```python
from build123d import *

# Parameters (mm, degrees)
F0_W         = 90
F0_H         = 11
F0_R         = 1.725
F0_R_2       = 1.7
F1_DEPTH     = 13
F2_R         = 5
F2_R_2       = 1.7
F3_DEPTH     = 24
F4_R         = 1.725
F5_DEPTH     = 24
F6_R         = 0.5
F7_DEPTH     = 12
F8_T1_DEPTH  = 28
F8_T6_DEPTH  = 105
F8_S7_R      = 5
F8_T8_DEPTH  = 54
F8_S9_R      = 5
F8_T10_DEPTH = 54
F8_T14_DEPTH = 105
F8_S15_R     = 5
F8_T16_DEPTH = 54
F8_S17_R     = 5
F8_T18_DEPTH = 54


# Not quite as in the source:
# - a fillet or chamfer that OpenCascade refuses, or shapes differently, is made with other operations: its cross-section is extruded or revolved along the edge and cut away or added
# - a feature names something its author has since deleted; it is built from what else it names


with BuildPart() as f1:
    # F0 (on Top) → F1 (new body)
    with BuildSketch(Plane.XY):
        Rectangle(F0_W, F0_H)
        with Locations((-40, 0)):
            Circle(F0_R, mode=Mode.SUBTRACT)
        with Locations((40, 0)):
            Circle(F0_R_2, mode=Mode.SUBTRACT)
    extrude(amount=F1_DEPTH)

    # F2 (on face) → F3 (join)
    with BuildSketch(Plane.XY.offset(13)):
        with Locations((40, 0)):
            Circle(F2_R)
        with Locations((40, 0)):
            Circle(F2_R_2, mode=Mode.SUBTRACT)
    extrude(amount=F3_DEPTH)

    # F4 (on face) → F5 (join)
    with BuildSketch(Plane.XY.offset(13)):
        with BuildLine():
            ThreePointArc((-45, 0), (-40, -5), (-35, 0))
            ThreePointArc((-35, 0), (-40, 5), (-45, 0))
        make_face()
        with Locations((-40, 0)):
            Circle(F4_R, mode=Mode.SUBTRACT)
    extrude(amount=F5_DEPTH)

    # F6 (on face) → F7 (cut)
    with BuildSketch(Plane.XY.offset(13)):
        with Locations((-20, 0)):
            Circle(F6_R)
        with Locations((20, 0)):
            Circle(F6_R)
    extrude(amount=-F7_DEPTH, mode=Mode.SUBTRACT)

    # F8: fillet of radius 3 on 6 edges, made by hand

    # F8_s2 → F8_t1 (cut)
    with BuildSketch(Plane.XY.offset(-7.5)):
        with BuildLine():
            ThreePointArc((-42, -5.5), (-44.1213203436, -4.6213203436), (-45, -2.5))
            Line((-45, -2.5), (-45, -5.5))
            Line((-45, -5.5), (-42, -5.5))
        make_face()
        with BuildLine():
            ThreePointArc((-45, 2.5), (-44.1213203436, 4.6213203436), (-42, 5.5))
            Line((-42, 5.5), (-45, 5.5))
            Line((-45, 5.5), (-45, 2.5))
        make_face()
        with BuildLine():
            ThreePointArc((42, -5.5), (44.1213203436, -4.6213203436), (45, -2.5))
            Line((45, -2.5), (45, -5.5))
            Line((45, -5.5), (42, -5.5))
        make_face()
        with BuildLine():
            ThreePointArc((45, 2.5), (44.1213203436, 4.6213203436), (42, 5.5))
            Line((42, 5.5), (45, 5.5))
            Line((45, 5.5), (45, 2.5))
        make_face()
    extrude(amount=F8_T1_DEPTH, mode=Mode.SUBTRACT)


with BuildPart() as f8_tool4:
    # F8_s5 → F8_t6 (new body)
    with BuildSketch(Plane.YZ.offset(-52.5)):
        with BuildLine():
            ThreePointArc((-5.5, 10), (-4.6213203436, 12.1213203436), (-2.5, 13))
            Line((-2.5, 13), (-5.5, 13))
            Line((-5.5, 13), (-5.5, 10))
        make_face()
    extrude(amount=F8_T6_DEPTH)

    # F8_s7 → F8_t8 (cut, symmetric)
    with BuildSketch(Plane.XY.offset(11.5)):
        with Locations((-40, 0)):
            Circle(F8_S7_R)
    extrude(amount=F8_T8_DEPTH, both=True, mode=Mode.SUBTRACT)

    # F8_s9 → F8_t10 (cut, symmetric)
    with BuildSketch(Plane.XY.offset(11.5)):
        with Locations((40, 0)):
            Circle(F8_S9_R)
    extrude(amount=F8_T10_DEPTH, both=True, mode=Mode.SUBTRACT)


with BuildPart() as f1_1:
    add(f1.part)

    # F8_t3: cut F8_tool4
    add(f8_tool4.part, mode=Mode.SUBTRACT)


with BuildPart() as f8_tool12:
    # F8_s13 → F8_t14 (new body)
    with BuildSketch(Plane.YZ.offset(52.5)):
        with BuildLine():
            ThreePointArc((2.5, 13), (4.6213203436, 12.1213203436), (5.5, 10))
            Line((5.5, 10), (5.5, 13))
            Line((5.5, 13), (2.5, 13))
        make_face()
    extrude(amount=-F8_T14_DEPTH)

    # F8_s15 → F8_t16 (cut, symmetric)
    with BuildSketch(Plane.XY.offset(11.5)):
        with Locations((-40, 0)):
            Circle(F8_S15_R)
    extrude(amount=F8_T16_DEPTH, both=True, mode=Mode.SUBTRACT)

    # F8_s17 → F8_t18 (cut, symmetric)
    with BuildSketch(Plane.XY.offset(11.5)):
        with Locations((40, 0)):
            Circle(F8_S17_R)
    extrude(amount=F8_T18_DEPTH, both=True, mode=Mode.SUBTRACT)


with BuildPart() as f1_2:
    add(f1_1.part)

    # F8_t11: cut F8_tool12
    add(f8_tool12.part, mode=Mode.SUBTRACT)

    # F9: fillet of radius 4 on 2 edges, made by hand

    # F9_s1 → F9_t2 (revolve, cut)
    with BuildSketch(Plane.XZ):
        with BuildLine():
            ThreePointArc((-38.275, 37), (-35.9259147702, 35.6255485658), (-35, 33.0662517874))
            Line((-35, 33.0662517874), (-35, 37))
            Line((-35, 37), (-38.275, 37))
        make_face()
    revolve(axis=Axis((-40, 0, 37), (0, 0, -1)), mode=Mode.SUBTRACT)

    # F9_s3 → F9_t4 (revolve, cut)
    with BuildSketch(Plane.XZ):
        with BuildLine():
            ThreePointArc((41.7, 37), (44.0659419434, 35.6307727822), (45, 33.0617262665))
            Line((45, 33.0617262665), (45, 37))
            Line((45, 37), (41.7, 37))
        make_face()
    revolve(axis=Axis((40, 0, 37), (0, 0, 1)), mode=Mode.SUBTRACT)


solid = f1_2.part
```
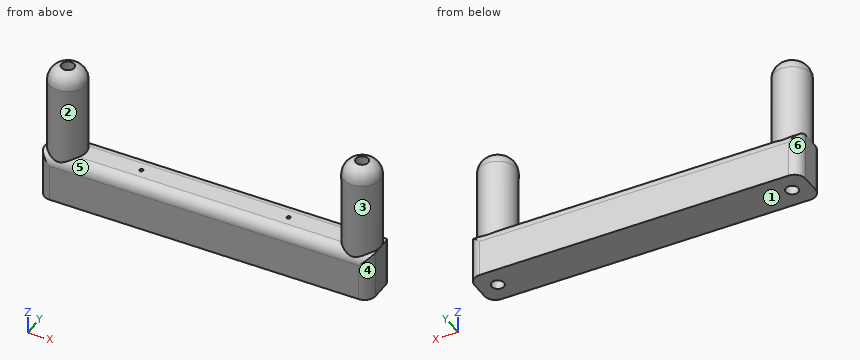
Build history of the part. All positions in model axes, mm. Face numbers are marked on the shaded views. A direction names the side the tool comes from. Round coordinates to 2 decimals unless told otherwise and drop trailing zeros. Order: outer loops, then holes, each group sorted by start corner. A loop starts at its lowest first (then second) coordinate and runs counter-clockwise, first axis right, second up. Notation, with made-up numbers: (56, 78) - (74, 78) arc R10 cw to (74, 93) - close; hole circle Ø11 at (69, 87.5). An arc over 180 degrees is marked (long way). Use a Markdown table: item, result.
1) Wall check: L1, parallel to Y at x = -40, z = 29.5 (3 decimals); L2, parallel to Y at x = -20, z = 8; L3, parallel to Z at x = 28.5, y = 0.5. Give the ranges that are in metal, low to high.
Recorded:
| item | result |
|---|---|
| L1 | y = -5 to -1.725, 1.725 to 5 |
| L2 | y = -5.5 to -0.5, 0.5 to 5.5 |
| L3 | z = 0 to 13 |
2) Saw through at A-A on z = 24. Write the cut outline in (x, y) (3 decimals), and give its area (3 significant figures).
Recorded:
| item | result |
|---|---|
| outline | circle Ø10 at (-40, 0); circle Ø10 at (40, 0); hole circle Ø3.45 at (-40, 0); hole circle Ø3.4 at (40, 0) |
| area | 139 mm² |
3) Flat gauge pins, fed straight in: pin 1 Ø2 at (x, y) = (-4.5, 0.5) entering from +Z; pin 2 Ø0.7 at (x, y) = (44.5, -1.5) entering from +Z; pin 3 Ø3 at (y, z) = (-3.5, 31) entering from -X. Where does each tip first touch, or does it go through?
Recorded:
| item | result |
|---|---|
| pin 1 | stops at z = 13 |
| pin 2 | stops at z = 35.18 |
| pin 3 | stops at x = -44.58 |
4) Pull direction X, two halves, no side cores. Call the marked faces 1, 2, 3 and 4: pulls with the +X half, pulls with the -X half, needs draft (parallel to the pull), parting line crosses it, or undercut.
Recorded:
| item | result |
|---|---|
| face 1 | needs draft |
| face 2 | undercut |
| face 3 | undercut |
| face 4 | pulls with the +X half |
5) Tool access for the marked faces 5 and 6: list every direction of +Z, -Z, +X, -X, +Y, -Y with a clear straight run to the whole face (end or side of a thin tool).
Recorded:
| item | result |
|---|---|
| face 5 | +Z, -Y |
| face 6 | +Z, -Z, -X, +Y |
6) Saw through at B-B on x = 15. Write the cut outline in (y, z).
Recorded:
| item | result |
|---|---|
| outline | (-5.5, 0) - (5.5, 0) - (5.5, 10) arc R3 ccw to (2.5, 13) - (-2.5, 13) arc R3 ccw to (-5.5, 10) - close |
